Autodesk Inventor part; units mm, degrees
ref_plane "YZ Plane" through (0, 0, 0) normal (1, 0, 0) x (0, 1, 0)
ref_plane "XZ Plane" through (0, 0, 0) normal (0, 1, 0) x (-1, 0, 0)
ref_plane "XY Plane" through (0, 0, 0) normal (0, 0, 1) x (1, 0, 0)
sketch "Sketch1" plane through (0, 0, 0) normal (0, 0, 1) x (1, 0, 0)
  line L0 (-56, 0) -> (-28, 48.4974)
  line L1 (-28, 48.4974) -> (28, 48.4974)
  line L2 (28, 48.4974) -> (56, 0)
  line L3 (56, 0) -> (28, -48.4974)
  line L4 (28, -48.4974) -> (-28, -48.4974)
  line L5 (-28, -48.4974) -> (-56, 0)
  line L6 (28, 48.4974) -> (86, 48.4974)
  line L7 (86, 48.4974) -> (86, -48.4974)
  line L8 (86, -48.4974) -> (28, -48.4974)
  point P0 (0, 0)
  point P1 (0, 0)
  dimension "d0" = 112
  dimension "d1" = 30
extrude "Extrusion1" add sketch "Sketch1" along normal blind 5
sketch "Sketch2" plane through (0, 0, 0) normal (0, 0, -1) x (-1, 0, 0)
  line L0 (-86, 48.4974) -> (28, 48.4974)
  line L1 (28, 48.4974) -> (56, 0)
  line L2 (56, 0) -> (28, -48.4974)
  line L3 (28, -48.4974) -> (-86, -48.4974)
  line L4 (-86, 33.4974) -> (19.3397, 33.4974)
  line L5 (19.3397, 33.4974) -> (38.6795, 0)
  line L6 (38.6795, 0) -> (19.3397, -33.4974)
  line L7 (19.3397, -33.4974) -> (-86, -33.4974)
  line L8 (-86, -48.4974) -> (-86, 48.4974)
  line L9 (-86, -48.4974) -> (-86, 48.4974)
  line L10 (-86, 48.4974) -> (-66, 48.4974)
  line L11 (-66, 48.4974) -> (-66, -48.4974)
  line L12 (-66, -48.4974) -> (-86, -48.4974)
  line L13 (-86, -48.4974) -> (-86, 48.4974)
  line L14 (-86, 48.4974) -> (-86, 33.4974)
  line L15 (-86, -33.4974) -> (-86, -48.4974)
  point P0 (0, 0)
  dimension "d4" = 15
  dimension "d5" = 20
extrude "Extrusion2" add sketch "Sketch2" along normal blind 15 contours L0 L11 L4 L8 | L0 L1 L2 L3 L11 L7 L6 L5 L4 | L4 L11 L7 L8 | L7 L11 L3 L8
sketch "Sketch3" plane through (0, 0, 5) normal (0, 0, 1) x (1, 0, 0)
  line L0 (86, 48.4974) -> (-28, 48.4974)
  line L1 (-28, 48.4974) -> (-56, 0)
  line L2 (-56, 0) -> (-28, -48.4974)
  line L3 (-28, -48.4974) -> (86, -48.4974)
  line L4 (86, -48.4974) -> (86, 48.4974)
  line L5 (76, -38.4974) -> (-22.2265, -38.4974)
  line L6 (-22.2265, -38.4974) -> (-44.453, 0)
  line L7 (-44.453, 0) -> (-22.2265, 38.4974)
  line L8 (-22.2265, 38.4974) -> (76, 38.4974)
  line L9 (76, 38.4974) -> (76, -38.4974)
  point P0 (0, 0)
  dimension "d8" = 10
extrude "Extrusion3" cut sketch "Sketch3" against normal through all
sketch "Sketch4" plane through (0, 0, 0) normal (0, 0, -1) x (-1, 0, 0)
  line L0 (-76, -38.4974) -> (-86, -38.4974)
  line L1 (-86, -38.4974) -> (-86, 38.4974)
  line L2 (-86, 38.4974) -> (-76, 38.4974)
  line L3 (-76, 38.4974) -> (-76, -38.4974)
  point P0 (0, 0)
  dimension "d11" = 10
extrude "Extrusion4" add sketch "Sketch4" along normal blind 15 and the other way blind 5
sketch "Sketch5" plane through (0, 0, 0) normal (0, 0, -1) x (-1, 0, 0)
  line L0 (-66, 33.4974) -> (-66, -33.4974)
  line L1 (-66, -33.4974) -> (19.3397, -33.4974)
  line L2 (19.3397, -33.4974) -> (38.6795, 0)
  line L3 (38.6795, 0) -> (19.3397, 33.4974)
  line L4 (19.3397, 33.4974) -> (-66, 33.4974)
  point P0 (0, 0)
extrude "Extrusion5" add sketch "Sketch5" along normal blind 5
sketch "Sketch7" plane through (0, 0, 5) normal (0, 0, 1) x (1, 0, 0)
  line L0 (86, 38.4974) -> (-22.2265, 38.4974)
  line L1 (-22.2265, 38.4974) -> (-44.453, 0)
  line L2 (-44.453, 0) -> (-22.2265, -38.4974)
  line L3 (-22.2265, -38.4974) -> (86, -38.4974)
  line L4 (86, -38.4974) -> (86, 38.4974)
  point P0 (0, 0)
extrude "Extrusion6" cut sketch "Sketch7" against normal blind 5
sketch "Sketch8" plane through (66, -33.4974, -15) normal (-1, 0, 0) x (0, 0, 1)
  line L0 (10, 0) -> (10, 66.9948)
  line L1 (0, 66.9948) -> (10, 66.9948)
  line L2 (0, 0) -> (0, 66.9948)
  line L3 (10, 0) -> (0, 0)
  line L4 (0, 71.9948) -> (0, -5)
  line L5 (0, 25.9974) -> (10, 25.9974)
  line L6 (10, 25.9974) -> (10, 40.9974)
  line L7 (10, 40.9974) -> (0, 40.9974)
  line L8 (0, 40.9974) -> (0, 25.9974)
  point P0 (15, 33.4974)
  point P1 (10, 33.4974)
  dimension "d20" = 15
extrude "Extrusion7" cut sketch "Sketch8" against normal through all contours L5 L2 L7 L0
sketch "Sketch9" plane through (0, 0, -15) normal (0, 0, -1) x (-1, 0, 0)
  line L0 (-86, -7.5) -> (-86, 7.5) construction
  line L1 (-66, -7.5) -> (-86, -7.5) construction
  line L2 (-78.5, -27.5) -> (-78.5, 27.5) construction
  circle A0 centre (-78.5, -27.5) radius 2.5
  circle A1 centre (-78.5, 27.5) radius 2.5
  point P0 (0, 0)
  point P1 (-78.5, 0)
  point P2 (-86, 0)
  dimension "d23" = 55
  dimension "d24" = 5
  dimension "d25" = 5
  dimension "d32" = 7.5
extrude "Extrusion8" cut sketch "Sketch9" against normal through all
sketch "Sketch10" plane through (0, 0, 0) normal (0, 0, 1) x (1, 0, 0)
  circle A0 centre (78.5, -27.5) radius 2.5
  circle A1 centre (78.5, 27.5) radius 2.5
  line L0 (-22.2265, 38.4974) -> (86, 38.4974)
  line L1 (-44.453, 0) -> (-22.2265, 38.4974)
  line L2 (-22.2265, -38.4974) -> (-44.453, 0)
  line L3 (86, -38.4974) -> (-22.2265, -38.4974)
  line L4 (86, 38.4974) -> (86, -38.4974)
  line L5 (-43.8756, 0) -> (-21.9378, 37.9974)
  line L6 (-21.9378, 37.9974) -> (85.5, 37.9974)
  line L7 (85.5, 37.9974) -> (85.5, -37.9974)
  line L8 (85.5, -37.9974) -> (-21.9378, -37.9974)
  line L9 (-21.9378, -37.9974) -> (-43.8756, 0)
  point P0 (0, 0)
  dimension "d29" = 0.5
extrude "Extrusion9" cut sketch "Sketch10" against normal through all contours L0 L4 L3 L2 L1
sketch "Sketch12" plane through (0, 0, -15) normal (0, 0, -1) x (-1, 0, 0)
  line L0 (-85.5, 37.9974) -> (-85.5, 7.5)
  line L1 (-85.5, 7.5) -> (-66, 7.5)
  line L2 (-66, 7.5) -> (-66, 33.4974)
  line L3 (-66, 33.4974) -> (19.3397, 33.4974)
  line L4 (19.3397, 33.4974) -> (38.6795, 0)
  line L5 (38.6795, 0) -> (19.3397, -33.4974)
  line L6 (19.3397, -33.4974) -> (-66, -33.4974)
  line L7 (-66, -33.4974) -> (-66, -7.5)
  line L8 (-66, -7.5) -> (-85.5, -7.5)
  line L9 (-85.5, -7.5) -> (-85.5, -37.9974)
  line L10 (-85.5, -37.9974) -> (21.9378, -37.9974)
  line L11 (21.9378, -37.9974) -> (43.8756, 0)
  line L12 (43.8756, 0) -> (21.9378, 37.9974)
  line L13 (21.9378, 37.9974) -> (-85.5, 37.9974)
  circle A0 centre (-78.5, -27.5) radius 2.5
  circle A1 centre (-78.5, 27.5) radius 2.5
  point P0 (0, 0)
extrude "Extrusion11" add sketch "Sketch12" along normal blind 10
sketch "Sketch13" plane through (85.5, -37.9974, 0) normal (1, 0, 0) x (0, 0, -1)
  line L0 (5, 45.4974) -> (5, 30.4974)
  line L1 (25, 45.4974) -> (5, 45.4974)
  line L2 (5, 45.4974) -> (15, 45.4974)
  line L3 (15, 45.4974) -> (15, 30.4974)
  line L4 (15, 30.4974) -> (5, 30.4974)
  line L5 (5, 30.4974) -> (5, 45.4974)
  line L6 (5, 30.4974) -> (25, 30.4974)
  point P0 (0, 37.9974)
  dimension "d39" = 10
extrude "Extrusion12" add sketch "Sketch13" against normal blind 19.5
properties part number "TARM05" material "ABS Plastic"
Could you check a few things on this model? Use its own coordinates, in mm. A direction names the side the tool comes from. Coordinates: 2 decimals unless noted, no trailing zeros. Loops run counter-clockwise (first coordinate to the right, second up) from the corner with the lowest first, then second, coordinate; pieces in that order, holes last.
1) Imagine slicing it at C-C (y = -27.5). List the corners of the cut face in (x, z) for me, and give its area (3 significant figures).
Reported:
outline: (-28, -25) - (-22.8, -25) - (-22.8, -5) - (66, -5) - (66, -25) - (76, -25) - (76, 0) - (-28, 0) - close; (81, -25) - (85.5, -25) - (85.5, 0) - (81, 0) - close
area: 936 mm2
2) Thinking about a two-plate mould opening in Y: for faces 4 (the face through (85.5, 1, -12)), 5 (the face through (-33.06, 18.73, -12.32)), 6 (the face through (33, -37.997, -12)), 7 (the face through (76, -7.5, -20)), which applies, released by +Y, released by -Y, zero draft, split by the parting line, or undercut?
Reported:
face 4: zero draft
face 5: released by +Y
face 6: released by -Y
face 7: undercut
3) Imagine slicing it at B-B (z = -1.75). List the corners of the cut face in (x, y) for me, and give its area (3 significant figures).
Reported:
outline: (-43.88, 0) - (-21.94, -38) - (85.5, -38) - (85.5, 38) - (-21.94, 38) - close; hole circle Ø5 at (78.5, -27.5); hole circle Ø5 at (78.5, 27.5)
area: 8,960 mm2
4) Imagine slicing it at D-D (z = -10.5). List the corners of the cut face in (x, y) for me.
Reported:
outline: (-43.88, 0) - (-21.94, -38) - (85.5, -38) - (85.5, 38) - (-21.94, 38) - close; hole (-38.68, 0) - (-19.34, -33.5) - (66, -33.5) - (66, 33.5) - (-19.34, 33.5) - close; hole circle Ø5 at (78.5, -27.5); hole circle Ø5 at (78.5, 27.5)
5) Will these pins go through, and if not, where does the flat tip stop? pin 1 Ø3 at (x, y) = (78.5, -27.5) entering from +Z; pin 2 Ø7.5 at (x, y) = (75, 2.5) entering from -Z; pin 3 Ø6 at (x, y) = (22, -15) entering from -Z; pin 4 Ø1.5 at (y, z) = (-0.5, -12.5) entering from -X.
Reported:
pin 1: passes through
pin 2: stops at z = -15
pin 3: stops at z = -5
pin 4: stops at x = -43.88
6) Which directions (+Z, -Z, +X, -X, +Y, -Y) give clear straight access to the entire face, cutting with the end or side of a thin tool? Please do faces 1 (the face through (23, -33.497, -15)), 2 (the face through (69, 9, -25)), 3 (the face through (76, 7.5, -20)).
Reported:
face 1: -Z
face 2: -Z, +X, -X, +Y, -Y
face 3: -Z, +X
7) Please list where these lines run through material, in increasing order: line 1 along Y through (x, z) = (78.5, -5.75); line 2 along Y through (x, z) = (78.5, -15.5); line 3 along Y through (x, z) = (-12.5, -9.5).
Reported:
line 1: y = -38 to -30, -25 to 25, 30 to 38
line 2: y = -38 to -30, -25 to -7.5, 7.5 to 25, 30 to 38
line 3: y = -38 to -33.5, 33.5 to 38
8) Imagine slicing it at A-A (x = 78.5). List the corners of the cut face in (y, z) for me, and give its area (3 significant figures).
Reported:
outline: (-38, -25) - (-30, -25) - (-30, 0) - (-38, 0) - close; (-25, -25) - (-7.5, -25) - (-7.5, -15) - (7.5, -15) - (7.5, -25) - (25, -25) - (25, 0) - (-25, 0) - close; (30, -25) - (38, -25) - (38, 0) - (30, 0) - close
area: 1,500 mm2
